Verification items for the finished model (mm, model axes). Coordinates: 2 decimals unless noted, no trailing zeros. Write each loop counter-clockwise with the first axis right and the second up, starting at its lowest first coordinate (ties: lowest second). Pieces come first, ordered by that corner, then holes. Notation, with made-up numbers: M -24,76.25 L 19,76.25 A28 cw 19,99.25 Z; hole C -13.75,55.25 d5. An arc over 180 degrees is marked long. Answer in a Markdown table with one row per item.
from build123d import *

# Parameters (mm, degrees)
SKETCH_4_W               = 180
SKETCH_4_H               = 180
EXTRUDE_1_DEPTH          = 1320
SKETCH_5_W               = 15
SKETCH_5_H               = 15
CUT_EXTRUDE_1_DEPTH      = 1320
CUT_EXTRUDE_2_DEPTH      = 1
CUT_EXTRUDE_2_DEPTH_BACK = 181
CUT_EXTRUDE_3_DEPTH      = 181
SKETCH_8_W               = 150
SKETCH_8_H               = 150
EXTRUDE_2_DEPTH          = 15


with BuildPart() as part:
    # 草图4 → 凸台-拉伸1 (new body)
    with BuildSketch(Plane(origin=(0, 0, 0), x_dir=(1, 0, 0), z_dir=(0, 1, 0))):
        with Locations((90, 90)):
            Rectangle(SKETCH_4_W, SKETCH_4_H)
    extrude(amount=-EXTRUDE_1_DEPTH)

    # 草图5 → 切除-拉伸1 (cut)
    with BuildSketch(Plane(origin=(0, 0, 0), x_dir=(1, 0, 0), z_dir=(0, 1, 0))):
        with Locations((7.5, 172.5)):
            Rectangle(SKETCH_5_W, SKETCH_5_H)
        with Locations((7.5, 7.5)):
            Rectangle(SKETCH_5_W, SKETCH_5_H)
        with Locations((172.5, 172.5)):
            Rectangle(SKETCH_5_W, SKETCH_5_H)
        with Locations((172.5, 7.5)):
            Rectangle(SKETCH_5_W, SKETCH_5_H)
    extrude(amount=-CUT_EXTRUDE_1_DEPTH, mode=Mode.SUBTRACT)

    # 草图6 → 切除-拉伸2 (cut, two sides)
    with BuildSketch(Plane.XY) as cut_extrude_2_sk:
        with BuildLine():
            Line((0, -200.607378165), (0, -249.392621835))
            ThreePointArc((0, -249.392621835), (17, -225), (0, -200.607378165))
        make_face()
        with BuildLine():
            Line((180, -200.607378165), (180, -249.392621835))
            ThreePointArc((180, -249.392621835), (163, -225), (180, -200.607378165))
        make_face()
    extrude(amount=CUT_EXTRUDE_2_DEPTH, mode=Mode.SUBTRACT)
    extrude(cut_extrude_2_sk.sketch, amount=-CUT_EXTRUDE_2_DEPTH_BACK, mode=Mode.SUBTRACT)

    # 草图7 → 切除-拉伸3 (cut, through all)
    with BuildSketch(Plane.ZY):
        with BuildLine():
            Line((-180, -200.607378165), (-180, -249.392621835))
            ThreePointArc((-180, -249.392621835), (-163, -225), (-180, -200.607378165))
        make_face()
        with BuildLine():
            Line((0, -200.607378165), (0, -249.392621835))
            ThreePointArc((0, -249.392621835), (-17, -225), (0, -200.607378165))
        make_face()
    extrude(amount=-CUT_EXTRUDE_3_DEPTH, mode=Mode.SUBTRACT)

    # 草图8 → 凸台-拉伸2 (add)
    with BuildSketch(Plane(origin=(0, 0, 0), x_dir=(1, 0, 0), z_dir=(0, 1, 0))):
        with Locations((90, 90)):
            Rectangle(SKETCH_8_W, SKETCH_8_H)
    extrude(amount=EXTRUDE_2_DEPTH)


solid = part.part
1) Release check for a two-part mould opening along Y. For faces 1 (the face through (89, -225, -163)), 2 (the face through (89, -1320, -91)), 3 (the face through (180, -777, -89)), 4 (the face through (163, -225, -89)) record: +Y half, -Y half, draft (parallel to the pull), parting line (faces both ways), or undercut.
Response values:
| item | result |
|---|---|
| face 1 | undercut |
| face 2 | -Y half |
| face 3 | draft |
| face 4 | undercut |
2) Sectioned sample at A-A (y = -1147.5). Record the cut outline in (x, z).
Response values:
| item | result |
|---|---|
| outline | M 0,-165 L 15,-165 L 15,-180 L 165,-180 L 165,-165 L 180,-165 L 180,-15 L 165,-15 L 165,0 L 15,0 L 15,-15 L 0,-15 Z |
3) Depth check by flat-ended pin: pin 1 (7.5 mm diameter, centred on y = -536.5, z = -172.5, fed in from +X); pin 2 (7.5 mm diameter, centred on x = 9, y = -127, fed in from +Z); pin 3 (4.5 mm diameter, centred on x = 173, z = -115.5, fed in from +Y). Enter the tip coordinate at first touch or a pass-through.
Response values:
| item | result |
|---|---|
| pin 1 | stops at x = 165 |
| pin 2 | stops at z = -15 |
| pin 3 | stops at y = 0 |
4) Thickness scan on L1, parallel to Z at x = 166.5, y = -1108. Record the ranges inside material, lowest first. Write a range as [from, to].
Response values:
| item | result |
|---|---|
| L1 | z = [-165, -15] |
